Study the drawing (mm; zero at the part's minimum x, y, z) and answer. Coordinates: 2 decimals unless noted, no trailing zeros. Loops run counter-clockwise (first coordinate to the right, second up) from the corner with the lowest first, then second, coordinate; pieces in that order, holes last. Notation, with made-up numbers: (-14, 76) - (6, 76) arc R28 cw to (6, 103) - close; hole circle Ø3 at (64.5, -9.5). An arc over 180 degrees is marked (long way). One line per item, written item: value. Start each with the question number.
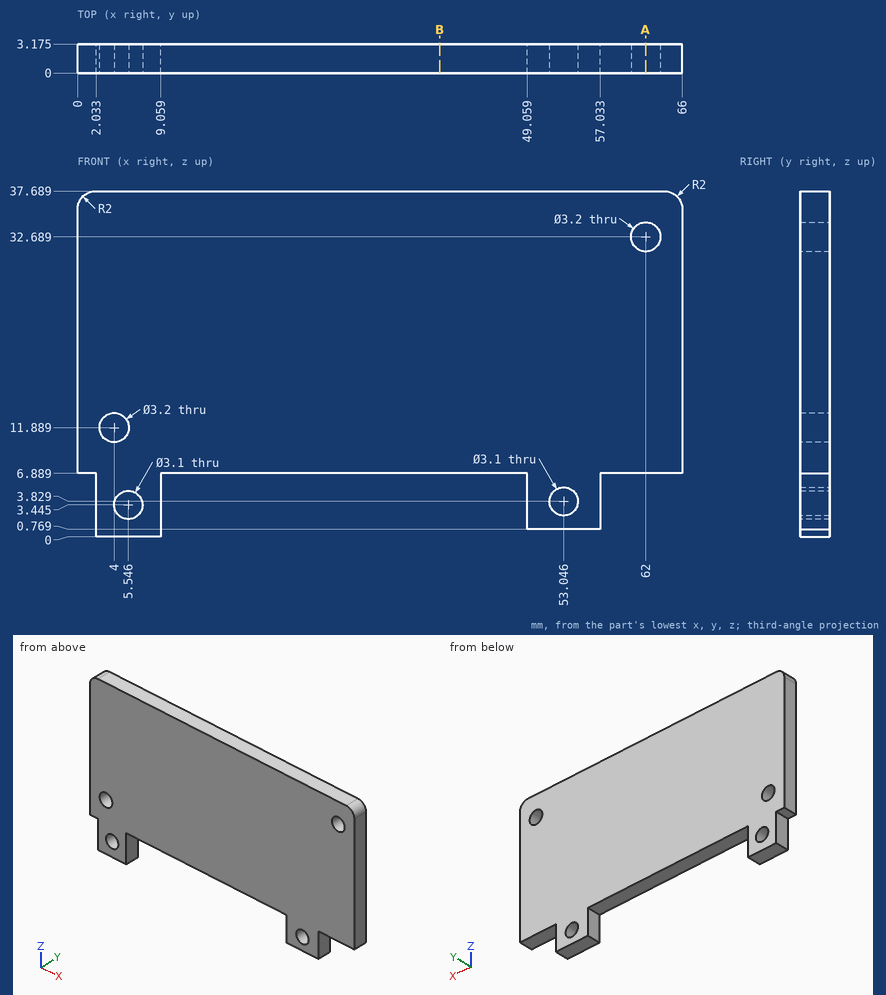
1) Section A-A, the plane x = 62 is taken. Determine the outline of the cut face in (y, z) (1 decimal).
2) Section B-B, the plane x = 39.5 is taken. Determine the outline of the cut face in (y, z) (1 decimal).
3) Straight lines are drawn through the part: L1, parallel to X at y = 1.9, z = 32.5; L2, parallel to X at y = 0.2, z = 4 (1 decimal); L3, parallel to Z at x = 54, y = 1.9. For each, find the intervals that lie inside material, in ascending order.
4) Flat-ended cylindrical pins translate along their axes: P1, Ø2.5, axis at x = 53.05, z = 3.83, coming from the +Y side; P2, Ø1, axis at x = 59.5, y = 2, coming from the -Z side; P3, Ø1, axis at y = 2, z = 2, coming from the +X side; P4, Ø3.5, axis at x = 4, z = 11.89, coming from the -Y side. Find the tip coordinate at first contact, or state that the pin passes through.
Answer below:
1. outline: (0, 6.9) - (3.2, 6.9) - (3.2, 31.1) - (0, 31.1) - close; (0, 34.3) - (3.2, 34.3) - (3.2, 37.7) - (0, 37.7) - close
2. outline: (0, 6.9) - (3.2, 6.9) - (3.2, 37.7) - (0, 37.7) - close
3. L1: 0 to 60.41, 63.59 to 66
3. L2: 2 to 4.1, 7 to 9.1, 49.1 to 51.5, 54.6 to 57
3. L3: 0.77 to 2.61, 5.05 to 37.69
4. P1: through
4. P2: z = 6.89
4. P3: x = 57.03
4. P4: y = 0
